Design review of the part built by this model. Coordinates are the model's own, in mm. Face numbers are marked on the shaded views. A direction names the side the tool comes from. Round coordinates to 2 decimals unless told otherwise and drop trailing zeros. Order: outer loops, then holes, each group sorted by start corner. A loop starts at its lowest first (then second) coordinate and runs counter-clockwise, first axis right, second up.
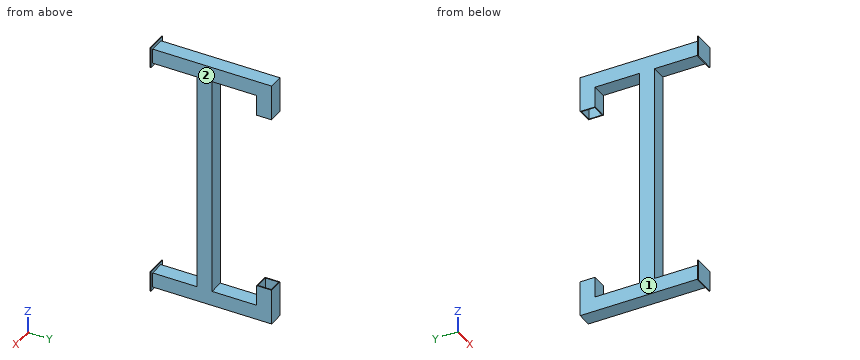
Autodesk Inventor part; units mm, degrees
ref_plane "YZ Plane" through (0, 0, 0) normal (1, 0, 0) x (0, 1, 0)
ref_plane "XZ Plane" through (0, 0, 0) normal (0, 1, 0) x (-1, 0, 0)
ref_plane "XY Plane" through (0, 0, 0) normal (0, 0, 1) x (1, 0, 0)
sketch "Boceto1" plane through (0, 0, 0) normal (0, 0, 1) x (1, 0, 0)
  line L0 (-15.875, -15.875) -> (15.875, -15.875)
  line L1 (15.875, -15.875) -> (15.875, 15.875)
  line L2 (15.875, 15.875) -> (-15.875, 15.875)
  line L3 (-15.875, 15.875) -> (-15.875, -15.875)
  line L4 (-15.875, -15.875) -> (15.875, 15.875) construction
  line L5 (15.875, -15.875) -> (-15.875, 15.875) construction
  line L6 (-17.875, 17.875) -> (17.875, 17.875)
  line L7 (17.875, 17.875) -> (17.875, -17.875)
  line L8 (17.875, -17.875) -> (-17.875, -17.875)
  line L9 (-17.875, -17.875) -> (-17.875, 17.875)
  point P0 (0, 0)
  dimension "d0" = 31.75
  dimension "d1" = 31.75
  dimension "d2" = 2
extrude "Extrusión1" add sketch "Boceto1" along normal mid plane 604
sketch "Boceto2" plane through (-17.875, -17.875, 302) normal (0, -1, 0) x (1, 0, 0)
  line L0 (0, 0) -> (35.75, 0)
  line L1 (0, 0) -> (35.75, 0)
  line L2 (35.75, 0) -> (35.75, -35.75)
  line L3 (35.75, -35.75) -> (0, -35.75)
  line L4 (0, -35.75) -> (0, 0)
  line L5 (33.75, -33.75) -> (33.75, -2)
  line L6 (33.75, -2) -> (2, -2)
  line L7 (2, -2) -> (2, -33.75)
  line L8 (2, -33.75) -> (33.75, -33.75)
  line L9 (35.75, -604) -> (35.75, 0)
  line L10 (0, -604) -> (35.75, -604)
  line L11 (35.75, -604) -> (35.75, -568.25)
  line L12 (35.75, -568.25) -> (0, -568.25)
  line L13 (0, -568.25) -> (0, -604)
  line L14 (33.75, -570.25) -> (33.75, -602)
  line L15 (33.75, -602) -> (2, -602)
  line L16 (2, -602) -> (2, -570.25)
  line L17 (2, -570.25) -> (33.75, -570.25)
  point P0 (17.875, -302)
  dimension "d5" = 35.75
  dimension "d6" = 35.75
  dimension "d7" = 2
extrude "Extrusión2" add sketch "Boceto2" along normal blind 250 and the other way blind 35.75
sketch "Boceto3" plane through (-17.875, -17.875, -266.25) normal (0, 0, 1) x (1, 0, 0)
  line L0 (35.75, 35.75) -> (35.75, -250)
  line L1 (35.75, -107.125) -> (0, -107.125)
  line L2 (0, -107.125) -> (0, -142.875)
  line L3 (0, -142.875) -> (35.75, -142.875)
  line L4 (35.75, -142.875) -> (35.75, -107.125)
  line L5 (2, -109.125) -> (33.75, -109.125)
  line L6 (33.75, -109.125) -> (33.75, -140.875)
  line L7 (33.75, -140.875) -> (2, -140.875)
  line L8 (2, -140.875) -> (2, -109.125)
  point P0 (17.875, 17.875)
  point P1 (35.75, -142.875)
  dimension "d12" = 35.75
  dimension "d13" = 35.75
  dimension "d14" = 2
extrude "Extrusión3" add sketch "Boceto3" along normal blind 532.5
sketch "Boceto4" plane through (-17.875, 17.875, 302) normal (0, 1, 0) x (1, 0, 0)
  line L0 (0, 568.25) -> (35.75, 568.25)
  line L1 (35.75, 604) -> (35.75, 0)
  line L2 (35.75, 518.25) -> (0, 518.25)
  line L3 (0, 604) -> (0, 0)
  line L4 (17.875, 302) -> (67.1432, 302)
  line L5 (35.75, 85.75) -> (0, 85.75)
  line L6 (0, 518.25) -> (0, 85.75)
  line L7 (35.75, 85.75) -> (35.75, 518.25)
  dimension "d17" = 50
extrude "Extrusión4" cut sketch "Boceto4" against normal blind 40 contours L2 L1 L5 L3
sketch "Boceto5" plane through (-17.875, -267.875, 302) normal (0, -1, 0) x (1, 0, 0)
  line L0 (33.75, -33.75) -> (33.75, -2)
  line L1 (33.75, -2) -> (2, -2)
  line L2 (-7.125, -42.875) -> (42.875, -42.875)
  line L3 (42.875, -42.875) -> (42.875, 7.125)
  line L4 (42.875, 7.125) -> (-7.125, 7.125)
  line L5 (-7.125, 7.125) -> (-7.125, -42.875)
  line L6 (-7.125, -42.875) -> (42.875, 7.125) construction
  line L7 (42.875, -42.875) -> (-7.125, 7.125) construction
  line L8 (-7.125, -561.125) -> (42.875, -561.125)
  line L9 (42.875, -561.125) -> (42.875, -611.125)
  line L10 (42.875, -611.125) -> (-7.125, -611.125)
  line L11 (-7.125, -611.125) -> (-7.125, -561.125)
  point P0 (17.875, -302)
  point P1 (17.875, -17.875)
  dimension "d20" = 50
  dimension "d21" = 50
extrude "Extrusión5" add sketch "Boceto5" along normal blind 2
sketch "Boceto6" plane through (-15.875, -15.875, -266.25) normal (0, 0, 1) x (1, 0, 0)
  line L0 (0, 31.75) -> (31.75, 31.75)
  line L1 (31.75, 31.75) -> (31.75, 0)
  line L2 (0, 31.75) -> (31.75, 31.75)
  line L3 (31.75, 31.75) -> (31.75, 0)
  line L4 (31.75, 0) -> (0, 0)
  line L5 (0, 0) -> (0, 31.75)
  point P0 (15.875, 15.875)
extrude "Extrusión6" cut sketch "Boceto6" along normal blind 550 and the other way blind 10
properties part number "Soporte_altura"
1) Take a section at D-D on x = 7. State how many separate pieces and enclosed holes the cut face has, plus the area to 3 significant figures.
Results:
separate pieces: 1
enclosed holes: 3
area: 5,140 mm2
2) Clearance check with flat-ended pins moving along their axes: P1, Ø16, axis at x = -1, y = -150.5, coming from the +Z side; P2, Ø2, axis at x = -1.5, z = -172, coming from the -Y side; P3, Ø4, axis at x = -1, y = -32, coming from the -Z side. State where each tip first meets the part, or that it passes through.
Results:
P1: stops at z = 302
P2: stops at y = -160.75
P3: stops at z = -302
3) Take a section at C-C on z = -38. Give the boundary of the cut face in (x, y) (3 decimals).
Results:
outline: (-17.875, -160.75) - (17.875, -160.75) - (17.875, -125) - (-17.875, -125) - close; hole (-15.875, -158.75) - (15.875, -158.75) - (15.875, -127) - (-15.875, -127) - close
4) To check wall thickness, follow line 1 along Z through (x, y) = (2, -79); line 2 along Y through (x, z) = (-14, 222) (3 decimals); line 3 along X through (y, z) = (-156, -169) (3 decimals). State the ranges of each line that lie inside material, in increasing order.
Results:
line 1: z = -302 to -300, -268.25 to -266.25, 266.25 to 268.25, 300 to 302
line 2: y = -160.75 to -158.75, -127 to -125, -17.875 to -15.875, 15.875 to 17.875
line 3: x = -17.875 to -15.875, 15.875 to 17.875
5) Take a section at B-B on y = -225.5. Give the boundary of the cut face in (x, z) (3 decimals), plus the area to 3 significant figures.
Results:
outline: (-17.875, -302) - (17.875, -302) - (17.875, -266.25) - (-17.875, -266.25) - close; (-17.875, 266.25) - (17.875, 266.25) - (17.875, 302) - (-17.875, 302) - close; hole (-15.875, -300) - (15.875, -300) - (15.875, -268.25) - (-15.875, -268.25) - close; hole (-15.875, 268.25) - (15.875, 268.25) - (15.875, 300) - (-15.875, 300) - close
area: 540 mm2
6) Take a section at A-A on z = -233.5. Give the boundary of the cut face in (x, y) (3 decimals), plus the area to 3 significant figures.
Results:
outline: (-17.875, -160.75) - (17.875, -160.75) - (17.875, -125) - (-17.875, -125) - close; (-17.875, -17.875) - (17.875, -17.875) - (17.875, 17.875) - (-17.875, 17.875) - close; hole (-15.875, -158.75) - (15.875, -158.75) - (15.875, -127) - (-15.875, -127) - close; hole (-15.875, -15.875) - (15.875, -15.875) - (15.875, 15.875) - (-15.875, 15.875) - close
area: 540 mm2
7) For the marked faces 1 and 2, list the 3-axis set-ups (+Z, -Z, +X, -X, +Y, -Y) from which the entire face can be reached by the end or side of a thin tool; tool diameter is ignored.
Results:
face 1: +Z, -Z, -X, +Y
face 2: +Z, -Z, +X, +Y
